Answer from the drawing. Dimensions are ordinates in mm from the lowest x, y and z of the part. Coordinates: 2 decimals unless noted, no trailing zeros. Write each loop counter-clockwise with the first axis right and the second up, starting at its lowest first coordinate (ties: lowest second). Pieces come first, ordered by that corner, then holes.
1) The part is cut by section B-B (z = 8.5). Determine the outline of the cut face in (x, y) (1 decimal).
2) Find the intervals of material crossed by line 1 (Z direction, x = 53, y = 28); line 2 (Y direction, x = 59, z = 14); line 3 (Y direction, x = 9, z = 6.5), in increasing order.
3) The part is cut by section A-A (y = 75). Determine the outline of the cut face in (x, z).
4) Each of these flat-tipped pins is pushed along its axis until it touches: pin 1 Ø1.5 at (x, y) = (46.5, 9) entering from +Z; pin 2 Ø2 at (x, z) = (63, 9.5) entering from +Y. Where does it stop, or does it pass through?
5) The part is cut by section C-C (x = 29.5). Determine the outline of the cut face in (y, z).
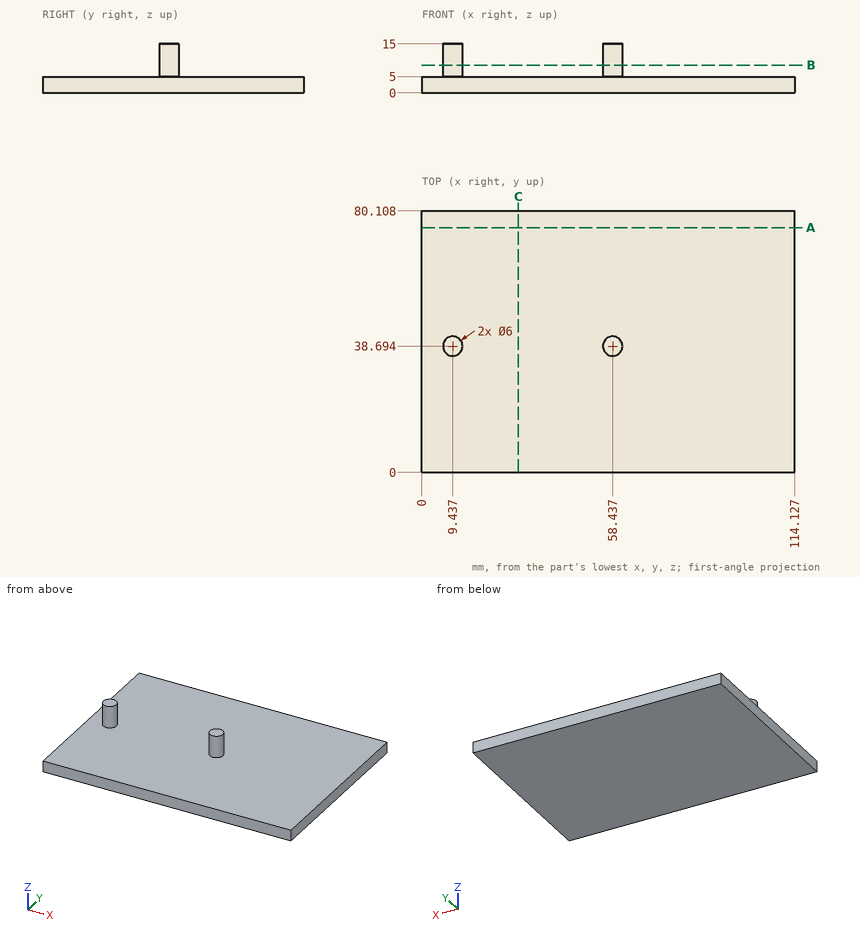
Reported:
1. outline: circle Ø6 at (9.4, 38.7); circle Ø6 at (58.4, 38.7)
2. line 1: z = 0 to 5
2. line 2: y = 35.75 to 41.64
2. line 3: y = 35.73 to 41.66
3. outline: (0, 0) - (114.13, 0) - (114.13, 5) - (0, 5) - close
4. pin 1: stops at z = 5
4. pin 2: passes through
5. outline: (0, 0) - (80.11, 0) - (80.11, 5) - (0, 5) - close
